For this review, take the finished solid that the model builds, in its own axes (mm). Face numbers are marked on the shaded views. A direction names the side the tool comes from. Round coordinates to 2 decimals unless told otherwise and drop trailing zeros. Order: outer loops, then holes, each group sorted by start corner. A loop starts at its lowest first (then second) coordinate and runs counter-clockwise, first axis right, second up. Notation, with made-up numbers: (37, 65.5) -> (72, 65.5) arc R32 cw to (72, 98.5) -> close; hole circle Ø1 at (5.5, 34.25). An arc over 180 degrees is marked (long way). Use a Markdown table: item, result. Add a question column.
1) Consider section B-B (z = 20.5). State the section outline as (x, y) points, plus the area to 3 significant figures.
2) Consider section A-A (y = -15). State the section outline as (x, z) points, plus the area to 3 significant figures.
3) Clearance check with flat-ended pins moving along their axes: P1, Ø8, axis at y = -70.5, z = 90.5, coming from the +X side; P2, Ø7.5, axis at y = -15, z = -65.48, coming from the +X side; P3, Ø10, axis at x = -24.5, z = 18, coming from the +Y side; P4, Ø1, axis at x = -36.5, y = -156.5, coming from the -Z side. State where each tip first meets the part, or that it passes through.
4) Consider section D-D (z = -43.5). State the section outline as (x, y) points, plus the area to 3 significant figures.
5) Machinability: for the marked faces 1, 2 and 3, which of the approach directions +Z, -Z, +X, -X, +Y, -Y give a long, thin tool a straight path to every point of the face, cutting with its end or side? Answer none if there is none.
6) Consider section C-C (x = -24). State the section outline as (y, z) points.
7) Wall thickness on line 1 along Z through (x, y) = (-49.5, -15); line 2 along Z through (x, y) = (35, -100); line 3 along X through (y, z) = (-139.5, 93): over which ranges is each line inside the solid? List them lowest first. Write a range as [from, to].
```python
from build123d import *

# Parameters (mm, degrees)
F1_DEPTH = 200
F2_W     = 10
F2_H     = 39.4300983846
F3_DEPTH = 70
F5_DEPTH = 70
F7_D     = 8.5


with BuildPart() as f1:
    # F0 (on Front) → F1 (new body)
    with BuildSketch(Plane.XZ):
        Polygon((-44.5507265627, 119.5215136588), (-54.5507265627, 119.5215136588), (-54.5507265627, -80.4784863412), (-44.5507265627, -80.4784863412), (-44.5507265627, 32.7215136588), (55.4492734373, 32.7215136588), (55.4492734373, 42.7215136588), (-44.5507265627, 42.7215136588), align=None)
    extrude(amount=F1_DEPTH)

    # F2 (on face) → F3 (join)
    with BuildSketch(Plane.YZ.offset(-44.5507265627)):
        with Locations((-100, 13.0064644665)):
            Rectangle(F2_W, F2_H)
    extrude(amount=F3_DEPTH)

    # F4 (on face) → F5 (cut)
    with BuildSketch(Plane(origin=(0, -95, 0), x_dir=(-1, 0, 0), z_dir=(0, 1, 0))):
        Polygon((44.5507265627, -6.7085847259), (-25.4492734373, 32.7215136588), (-25.4492734373, -6.7085847259), align=None)
    extrude(amount=-F5_DEPTH, mode=Mode.SUBTRACT)

    # F7 (through all)
    with Locations(Plane(origin=(-54.5507265627, 0, 0), x_dir=(0, -1, 0), z_dir=(-1, 0, 0))):
        with Locations((185, 104.5215136588), (15, 104.5215136588), (15, -65.4784863412), (185, -65.4784863412)):
            Hole(F7_D / 2)


solid = f1.part
```
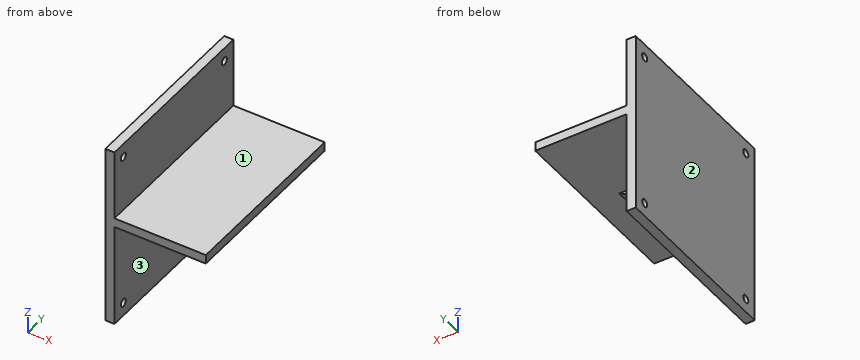
Results list:
| question | item | result |
|---|---|---|
| 1 | outline | (-54.55, -200) -> (-44.55, -200) -> (-44.55, -105) -> (3.75, -105) -> (3.75, -95) -> (-44.55, -95) -> (-44.55, 0) -> (-54.55, 0) -> close |
| 1 | area | 2,480 mm2 |
| 2 | outline | (-54.55, -80.48) -> (-44.55, -80.48) -> (-44.55, -69.73) -> (-54.55, -69.73) -> close; (-54.55, -61.23) -> (-44.55, -61.23) -> (-44.55, 32.72) -> (55.45, 32.72) -> (55.45, 42.72) -> (-44.55, 42.72) -> (-44.55, 100.27) -> (-54.55, 100.27) -> close; (-54.55, 108.77) -> (-44.55, 108.77) -> (-44.55, 119.52) -> (-54.55, 119.52) -> close |
| 2 | area | 2,830 mm2 |
| 3 | P1 | x = -44.55 |
| 3 | P2 | through |
| 3 | P3 | y = -95 |
| 3 | P4 | z = 32.72 |
| 4 | outline | (-54.55, -200) -> (-44.55, -200) -> (-44.55, 0) -> (-54.55, 0) -> close |
| 4 | area | 2,000 mm2 |
| 5 | face 1 | +Z, +X, +Y, -Y |
| 5 | face 2 | +Z, -Z, -X, +Y, -Y |
| 5 | face 3 | -Z, +X |
| 6 | outline | (-200, 32.72) -> (-105, 32.72) -> (-105, 4.87) -> (-95, 4.87) -> (-95, 32.72) -> (0, 32.72) -> (0, 42.72) -> (-200, 42.72) -> close |
| 7 | line 1 | [-80.48, -69.73], [-61.23, 100.27], [108.77, 119.52] |
| 7 | line 2 | [32.72, 42.72] |
| 7 | line 3 | [-54.55, -44.55] |
